Work out the finished part from the listing and answer in its coordinate system (mm). A direction names the side the tool comes from. Give positions to 0.01 mm unless a question says otherwise; leave off trailing zeros. Loops run counter-clockwise (first coordinate to the right, second up) from the corner with the lowest first, then second, coordinate; pieces in that order, holes last.
```python
from build123d import *

# Parameters (mm, degrees)
BOSS_EXTRUDE1_DEPTH = 15.9
SKETCH2_R           = 2.4
BOSS_EXTRUDE2_DEPTH = 1.8
LPATTERN1_COUNT     = 4
LPATTERN1_PITCH     = 8
SHELL1_T            = -1.2
SKETCH3_R           = 3.25
SKETCH3_R_2         = 2.4
BOSS_EXTRUDE3_DEPTH = 6.75
LPATTERN3_COUNT     = 2
LPATTERN3_PITCH     = 8
LPATTERN3_COL_COUNT = 2
LPATTERN3_COL_PITCH = 8
SKETCH4_W           = 9.930005036
SKETCH4_H           = 31.8
CUT_EXTRUDE1_DEPTH  = 21.430775863


with BuildPart() as part:
    # Sketch1 → Boss-Extrude1 (new, symmetric)
    with BuildSketch(Plane.XY):
        Polygon((0, 0), (-15.9, 0), (-15.9, 2), (-7.95, 7.95), (0, 7.95), align=None)
    extrude(amount=BOSS_EXTRUDE1_DEPTH, both=True)

    # Sketch2 → Boss-Extrude2 (add)
    with BuildSketch(Plane(origin=(0, 7.95, 0), x_dir=(1, 0, 0), z_dir=(0, 1, 0))):
        with Locations(Location((-4.05, -12, 0), (0, 0, 270))):
            Circle(SKETCH2_R)
    boss_extrude2 = extrude(amount=BOSS_EXTRUDE2_DEPTH)

    # LPattern1: Boss-Extrude2 ×4
    with Locations(*[(0, 0, -i * LPATTERN1_PITCH) for i in range(1, LPATTERN1_COUNT)]):
        add(boss_extrude2)

    # Shell1
    shell1_openings = [part.faces().sort_by_distance(p)[0] for p in [
        (-7.95, 0, 0),
    ]]
    offset(amount=SHELL1_T, openings=shell1_openings, kind=Kind.INTERSECTION)

    # Sketch3 → Boss-Extrude3 (add)
    with BuildSketch(Plane.XZ.offset(-6.75)):
        with Locations(Location((-8.015401462, 0, 0), (0, 0, 81.778871815))):
            Circle(SKETCH3_R)
        with Locations(Location((-8.015401462, 0, 0), (0, 0, 78.834853806))):
            Circle(SKETCH3_R_2, mode=Mode.SUBTRACT)
    boss_extrude3 = extrude(amount=BOSS_EXTRUDE3_DEPTH)

    # LPattern3: Boss-Extrude3 ×2
    with Locations(*[(0, 0, -i * LPATTERN3_PITCH) for i in range(1, LPATTERN3_COUNT)]):
        add(boss_extrude3)

    # LPattern3 col: Boss-Extrude3 ×2
    with Locations(*[(0, 0, i * LPATTERN3_COL_PITCH) for i in range(1, LPATTERN3_COL_COUNT)]):
        add(boss_extrude3)

    # Sketch4 → Cut-Extrude1 (cut, through all)
    with BuildSketch(Plane(origin=(-6.668067035, 8.909434106, 0), x_dir=(0.8006038236418165, 0.5991940566879009, 0), z_dir=(-0.5991940566879009, 0.8006038236418165, 0))):
        with Locations((-6.566210165, 0)):
            Rectangle(SKETCH4_W, SKETCH4_H)
    extrude(amount=CUT_EXTRUDE1_DEPTH, mode=Mode.SUBTRACT)


solid = part.part
```
Q1. Which of the six approach directions +Z, -Z, +X, -X, +Y, -Y give full straight-line access (tool end or side, diameter ignored) to faces 4 (the face through (-4.947, 2.672, 9.072)), 5 (the face through (-6.393, 8.837, 11.48)), 6 (the face through (-4, 9.75, -4))?
Q2. Determine the mould class of faces 1 (the face through (-4, 7.6, 2.8)), 2 (the face through (-6, 4, -15.9)), 3 (the face through (0, 4, 0)) for opening direction Z: +Z half, -Z half, draft (parallel to the pull), parting line (faces both ways), or undercut.
Q3. Given pin 1 (0.6 mm diameter, centred on x = -6.5, z = 8, fed in from -Y); pin 2 (0.7 mm diameter, centred on x = -4, z = -12, fed in from -Y); pin 3 (2 mm diameter, centred on x = -7, z = 0.5, fed in from -Y), each flat-ended and moving along its own axis, determine where each tip first touches the part or whether it passes through.
Q4. Section D-D on y = 9 is taken. Give the vertices of the cut face in (x, z), plus the area to 3 significant figures.
Q5. Section A-A on y = 6 is taken. Give the vertices of the cut face in (x, z), plus the area to 3 significant figures.
Q6. Section B-B on z = -4 is taken. Give the vertices of the cut face in (x, y), plus the area to 3 significant figures.
Q7. Consider line 1 along Z through (x, y) = (-4.05, 7.8); line 2 along X through (y, z) = (4.5, -8); line 3 along Z through (x, y) = (-1.25, 5). Determine where each line is inside the solid, lowest interval first.
Check result:
1. face 4: -Y
1. face 5: +Y
1. face 6: +Z, -Z, +X, -X, +Y
2. face 1: undercut
2. face 2: -Z half
2. face 3: draft
3. pin 1: stops at y = 6.75
3. pin 2: stops at y = 8.55
3. pin 3: stops at y = 6.41
4. outline: circle Ø4.8 at (-4.05, -12); circle Ø4.8 at (-4.05, -4); circle Ø4.8 at (-4.05, 4); circle Ø4.8 at (-4.05, 12)
4. area: 72.4 mm2
5. outline: (-10.56, -15.9) - (0, -15.9) - (0, 15.9) - (-10.56, 15.9) - close; hole (-8.55, -14.7) - (-1.2, -14.7) - (-1.2, 14.7) - (-8.55, 14.7) - (-8.55, 11.21) arc R3.25 cw (long way) to (-8.55, 4.79) - (-8.55, 3.21) arc R3.25 cw (long way) to (-8.55, -3.21) - (-8.55, -4.79) arc R3.25 cw (long way) to (-8.55, -11.21) - close; hole (-8.55, -10.34) arc R2.4 ccw (long way) to (-8.55, -5.66) - close; hole (-8.55, -2.34) arc R2.4 ccw (long way) to (-8.55, 2.34) - close; hole (-8.55, 5.66) arc R2.4 ccw (long way) to (-8.55, 10.34) - close
5. area: 145 mm2
6. outline: (-15.9, 0) - (-14.7, 0) - (-14.7, 1.4) - (-7.55, 6.75) - (-5.25, 6.75) - (-5.25, 8.55) - (-2.85, 8.55) - (-2.85, 6.75) - (-1.2, 6.75) - (-1.2, 0) - (0, 0) - (0, 7.95) - (-1.65, 7.95) - (-1.65, 9.75) - (-6.45, 9.75) - (-6.45, 7.95) - (-7.95, 7.95) - (-15.9, 2) - close
6. area: 35.1 mm2
7. line 1: z = -15.9 to -13.2, -10.8 to -5.2, -2.8 to 2.8, 5.2 to 10.8, 13.2 to 15.9
7. line 2: x = -12.56 to -10.42, -5.62 to -4.77, -1.2 to 0
7. line 3: z = -15.9 to -14.7, 14.7 to 15.9
